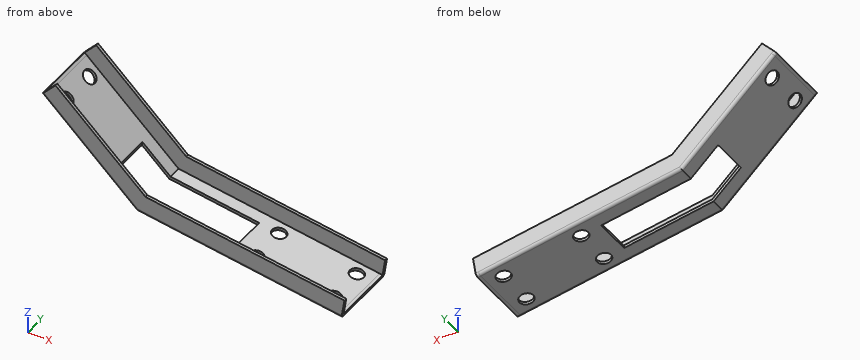
```python
from build123d import *

# Parameters (mm, degrees)
BOSS_EXTRUDE1_DEPTH = 26.64
BOSS_EXTRUDE2_DEPTH = 1.25
BOSS_EXTRUDE3_DEPTH = 1.25
FILLET1_R           = 1.25
SKETCH4_R           = 3
CUT_EXTRUDE1_DEPTH  = 1.25
BOSS_EXTRUDE4_START = 1.25
BOSS_EXTRUDE4_DEPTH = 1.25
SKETCH6_R           = 3
CUT_EXTRUDE2_DEPTH  = 1.25
BOSS_EXTRUDE5_DEPTH = 1.25
SKETCH8_W           = 51.440869123
SKETCH8_H           = 15.64
CUT_EXTRUDE3_DEPTH  = 21.25


with BuildPart() as part:
    # Sketch1 → Boss-Extrude1 (new body)
    with BuildSketch(Plane(origin=(0, 0, 0), x_dir=(1, 0, 0), z_dir=(0, 1, 0))):
        Polygon((83.457182963, 20.606052526), (-1.816223719, 7.555013068), (-40.71695424, -28.343507726), (-41.564678823, -27.424887548), (-2.383097929, 8.732808661), (83.268073317, 21.841664739), align=None)
    extrude(amount=BOSS_EXTRUDE1_DEPTH)

    # Sketch2 → Boss-Extrude2 (add)
    with BuildSketch(Plane(origin=(0, 26.64, 0), x_dir=(1, 0, 0), z_dir=(0, 1, 0))):
        Polygon((83.268073317, 21.841664739), (84.55401891, 13.439501688), (1.471646699, 0.723798632), (-35.800151659, -33.671504758), (-41.564678823, -27.424887548), (-2.383097929, 8.732808661), align=None)
    extrude(amount=BOSS_EXTRUDE2_DEPTH)

    # Sketch3 → Boss-Extrude3 (add)
    with BuildSketch(Plane.XZ):
        Polygon((83.268073317, -21.841664739), (84.55401891, -13.439501688), (1.471646699, -0.723798632), (-35.800151659, 33.671504758), (-41.564678823, 27.424887548), (-2.383097929, -8.732808661), align=None)
    extrude(amount=BOSS_EXTRUDE3_DEPTH)

    # Fillet1
    fillet1_edges = [part.edges().sort_by_distance(p)[0] for p in [
        (40.442487694, 27.89, -15.2872367),
        (-21.973888376, 27.89, 9.346039443),
        (40.442487694, -1.25, -15.2872367),
        (-21.973888376, -1.25, 9.346039443),
    ]]
    fillet(fillet1_edges, radius=FILLET1_R)

    # Sketch4 → Cut-Extrude1 (cut)
    with BuildSketch(Plane(origin=(-1.360504034, 0, -8.889315992), x_dir=(-0.98848977068378, 0, 0.15128771679659964), z_dir=(-0.15128771679659964, 0, -0.98848977068378))):
        with Locations((-79.264014288, 21.14)):
            Circle(SKETCH4_R)
        with Locations((-45.964014288, 21.14)):
            Circle(SKETCH4_R)
        with Locations((-45.964014288, 5.5)):
            Circle(SKETCH4_R)
        with Locations((-79.264014288, 5.5)):
            Circle(SKETCH4_R)
    extrude(amount=-CUT_EXTRUDE1_DEPTH, mode=Mode.SUBTRACT)

    # Sketch5 → Boss-Extrude4 (add)
    with BuildSketch(Plane(origin=(84.628577351, 0, -12.952348747), x_dir=(-0.15128771679660272, 0, -0.9884897706837796), z_dir=(0.9884897706837796, 0, -0.15128771679660272)).offset(BOSS_EXTRUDE4_START)):
        with BuildLine():
            Line((0.492825475, -1.25), (7.742825475, -1.25))
            ThreePointArc((7.742825475, -1.25), (8.626708952, -0.883883476), (8.992825475, 0))
            Line((8.992825475, 0), (8.992825475, 26.64))
            ThreePointArc((8.992825475, 26.64), (8.626708952, 27.523883476), (7.742825475, 27.89))
            Line((7.742825475, 27.89), (0.492825475, 27.89))
            Line((0.492825475, 27.89), (0.492825475, 26.64))
            Line((0.492825475, 26.64), (7.742825475, 26.64))
            Line((7.742825475, 26.64), (7.742825475, 0))
            Line((7.742825475, 0), (0.492825475, 0))
            Line((0.492825475, 0), (0.492825475, -1.25))
        make_face()
    extrude(amount=-BOSS_EXTRUDE4_DEPTH)

    # Sketch6 → Cut-Extrude2 (cut)
    with BuildSketch(Plane(origin=(-5.448411315, 0, -5.904064448), x_dir=(-0.7348961423682216, 0, 0.6781796664102415), z_dir=(-0.6781796664102415, 0, -0.7348961423682216))):
        with Locations((42.794723214, 5.5)):
            Circle(SKETCH6_R)
        with Locations((42.794723214, 21.14)):
            Circle(SKETCH6_R)
    extrude(amount=-CUT_EXTRUDE2_DEPTH, mode=Mode.SUBTRACT)

    # Sketch7 → Boss-Extrude5 (add)
    with BuildSketch(Plane(origin=(-36.116267508, 0, 33.328951995), x_dir=(0.6781796664102416, 0, 0.7348961423682215), z_dir=(-0.7348961423682215, 0, 0.6781796664102416))):
        with BuildLine():
            Line((-8.033875955, 26.64), (-8.033875955, 0))
            ThreePointArc((-8.033875955, 0), (-7.667759432, -0.883883476), (-6.783875955, -1.25))
            Line((-6.783875955, -1.25), (0.466124045, -1.25))
            Line((0.466124045, -1.25), (0.466124045, 0))
            Line((0.466124045, 0), (-6.783875955, 0))
            Line((-6.783875955, 0), (-6.783875955, 26.64))
            Line((-6.783875955, 26.64), (0.466124045, 26.64))
            Line((0.466124045, 26.64), (0.466124045, 27.89))
            Line((0.466124045, 27.89), (-6.783875955, 27.89))
            ThreePointArc((-6.783875955, 27.89), (-7.667759432, 27.523883476), (-8.033875955, 26.64))
        make_face()
    extrude(amount=BOSS_EXTRUDE5_DEPTH)

    # Sketch8 → Cut-Extrude3 (cut)
    with BuildSketch(Plane(origin=(-1.360504034, 0, -8.889315992), x_dir=(-0.98848977068378, 0, 0.15128771679659964), z_dir=(-0.15128771679659964, 0, -0.98848977068378))):
        with Locations((-11.673373202, 13.32)):
            Rectangle(SKETCH8_W, SKETCH8_H)
    extrude(amount=-CUT_EXTRUDE3_DEPTH, mode=Mode.SUBTRACT)


solid = part.part
```
Input: part model. Units: mm. Frame: model coordinates. Give positions to 0.01 mm unless a question says otherwise; leave off trailing zeros. Write each loop counter-clockwise with the first axis right and the second up, starting at its lowest first coordinate (ties: lowest second). Pieces come first, ordered by that corner, then holes. Notation, with made-up numbers: (14, -29.5) - (63, -29.5) arc R30 cw to (63, 4.5) - close; hole circle Ø7 at (-21.75, 6.25). An arc over 180 degrees is marked (long way). Write item = value, one per line. Start each with the question number.
1) Material intervals for L1, parallel to Y at x = -25, z = 17.5; L2, parallel to X at y = 1, z = 7, sorted ascending. Write a range as [from, to].
2) Pin query (flat end, axial travel): pin 1 (6 mm diameter, centred on x = 51.5, y = 13.5, fed in from +Z); pin 2 (2 mm diameter, centred on x = -25, y = 17, fed in from -Z); pin 3 (1 mm diameter, centred on y = 17.5, z = -13, fed in from -X). Return the tip coordinate at first contact, or that it passes through.
3) Cut plane A-A (y = 16). Return loops of the section in (x, z), and give its area (3 significant figures).
4) Cut plane B-B (y = 4). Return loops of the section in (x, z).
Answers follow:
q1.L1 = [-1.25, 0], [26.64, 27.89]
q1.L2 = [-19.43, -17.59]
q2.pin_1 = -15.26
q2.pin_2 = 11.22
q2.pin_3 = 35.76
q3.outline = (-42.48, 28.27) - (-13.92, 1.91) - (-13.69, 3.4) - (-41.64, 29.19) - close; (35.6, -14.55) - (84.5, -22.03) - (84.69, -20.8) - (35.79, -13.31) - close
q3.area = 110 mm^2
q4.outline = (-42.48, 28.27) - (-38.81, 24.88) - (-37.96, 25.8) - (-41.64, 29.19) - close; (-34.99, 21.36) - (-2.38, -8.73) - (41.51, -15.45) - (41.7, -14.21) - (-1.82, -7.56) - (-34.14, 22.28) - close; (46.64, -16.24) - (74.42, -20.49) - (74.61, -19.25) - (46.83, -15) - close; (79.56, -21.27) - (84.5, -22.03) - (84.69, -20.8) - (79.75, -20.04) - close
